Could you check a few things on this model? Use its own coordinates, in mm. A direction names the side the tool comes from. Coordinates: 2 decimals unless noted, no trailing zeros. Order: outer loops, then holes, each group sorted by start corner. A loop starts at its lowest first (then second) coordinate and runs counter-clockwise, first axis right, second up.
```python
from build123d import *

# Parameters (mm, degrees)
F1_DEPTH = 127


with BuildPart() as f1:
    # F0 (on Front) → F1 (new body)
    with BuildSketch(Plane.XZ):
        Polygon((-23.368, 0), (17.907, 0), (21.082, 0), (21.082, 3.175), (17.907, 3.175), (17.907, 19.05), (11.557, 19.05), (11.557, 11.7475), (14.732, 11.7475), (14.732, 8.5725), (11.557, 8.5725), (11.557, 6.604), (8.89, 6.604), (8.89, 3.175), (-8.89, 3.175), (-8.89, 6.604), (-13.843, 6.604), (-13.843, 8.5725), (-17.018, 8.5725), (-17.018, 11.7475), (-13.843, 11.7475), (-13.843, 19.05), (-20.193, 19.05), (-20.193, 3.175), (-23.368, 3.175), align=None)
    extrude(amount=-F1_DEPTH)


solid = f1.part
```
Item 1: For pin 1 Ø2 at (y, z) = (60.5, 16) entering from -X; pin 2 Ø1 at (y, z) = (95.5, 6.5) entering from +X; pin 3 Ø1.5 at (x, y) = (-12, 59) entering from +Z, each with a flat end and sliding along its axis, tell me the tip position at first contact or that it passes through.
Item 2: I need wall thicknesses on line 1 (X direction, y = 102.5, z = 6); line 2 (Z direction, x = 13.5, y = 22.5); line 3 (X direction, y = 31.5, z = 16.75). Which ranges of each line are inside material? Lowest first, please.
Item 3: Suppose I cut it at D-D (x = -2). List the corners of the cut face in (y, z) for me (3 decimals), and give its area (3 significant figures).
Item 4: Thinking about a two-plate mould opening in Z: for faces 1 (the face through (0, 63, 3.175)), 2 (the face through (14.732, 63, 10)), 3 (the face through (8.89, 63, 5)), which applies, +Z half, -Z half, draft (parallel to the pull), parting line (faces both ways), or undercut?
Item 5: Which directions (+Z, -Z, +X, -X, +Y, -Y) give clear straight access to the entire face, cutting with the end or side of a thin tool? Please do faces 4 (the face through (-17.018, 63, 10)), 5 (the face through (-22, 63, 3.175)), 6 (the face through (20, 63, 3.175)), 7 (the face through (-13.843, 63, 15)).
Item 6: Suppose I cut it at A-A (z = 14). List the corners of the cut face in (x, y) for me.
Item 7: Suppose I cut it at C-C (x = -12.5). List the corners of the cut face in (y, z) for me.
Geometry results:
1. pin 1: stops at x = -20.19
1. pin 2: stops at x = 17.91
1. pin 3: stops at z = 6.6
2. line 1: x = -20.19 to -8.89, 8.89 to 17.91
2. line 2: z = 0 to 8.57, 11.75 to 19.05
2. line 3: x = -20.19 to -13.84, 11.56 to 17.91
3. outline: (0, 0) - (127, 0) - (127, 3.175) - (0, 3.175) - close
3. area: 403 mm2
4. face 1: +Z half
4. face 2: undercut
4. face 3: draft
5. face 4: +Y, -Y
5. face 5: +Z, -X, +Y, -Y
5. face 6: +Z, +X, +Y, -Y
5. face 7: +Z, +Y, -Y
6. outline: (-20.19, 0) - (-13.84, 0) - (-13.84, 127) - (-20.19, 127) - close; (11.56, 0) - (17.91, 0) - (17.91, 127) - (11.56, 127) - close
7. outline: (0, 0) - (127, 0) - (127, 6.6) - (0, 6.6) - close
